Verification items for the finished model (mm, model axes). Round coordinates to 2 decimals unless told otherwise and drop trailing zeros. Loops run counter-clockwise (first coordinate to the right, second up) from the corner with the lowest first, then second, coordinate; pieces in that order, holes last. Notation, with made-up numbers: M 29.5,74 L 63.5,74 A28 cw 63.5,102 Z; hole C 29.5,34 d8. An arc over 180 degrees is marked long. One line per item, written item: value.
Autodesk Fusion 360 part; units mm, degrees
sketch "Sketch1" plane through (0, 0, 0) normal (0, 0, 1) x (1, 0, 0)
  circle A0 centre (0, 0) radius 200
  dimension "d1" = 400
extrude "Extrude1" add sketch "Sketch1" along normal blind 250
sketch "Sketch2" plane through (0, 0, 250) normal (0, 0, 1) x (-1, 0, 0)
  circle A0 centre (0, 0) radius 200
  circle A1 centre (0, 0) radius 25
  dimension "d4" = 50
extrude "Extrude2" cut sketch "Sketch2" against normal blind 75 contours A1
fillet "Fillet1" radius 25 1 edges at (-186.4655, -72.3231, 250)
scale "Scale1" factor 2.5 about (0, 0, 0) bodies 1
(1) Mould release check, pull along Y, two halves, no side actions. Record for faces 1 (the face through (91, 6, 625)), 2 (the face through (1, -1, 437.5)), 3 (the face through (62.44, -2.75, 532.56)), 4 (the face through (-499.516, -21.984, 277.312)): +Y half, -Y half, draft (parallel to the pull), parting line (faces both ways), or undercut.
Completed:
face 1: draft
face 2: undercut
face 3: undercut
face 4: parting line
(2) Thickness scan on L1, parallel to Y at x = 0, z = 486.5; L2, parallel to Y at x = 0, z = 433; L3, parallel to Z at x = -272, y = -344.5. Record the ranges inside material, lowest first. Write a range as from..to.
Completed:
L1: y = -500..-62.5, 62.5..500
L2: y = -500..500
L3: z = 0..624.98
(3) Sectioned sample at C-C on z = 205. Enter the section's corners in (x, y), and give its area (3 significant figures).
Completed:
outline: C 0,0 d1000
area: 785,000 mm^2
(4) Sectioned sample at A-A on x = 0. Enter the section's corners in (y, z).
Completed:
outline: M -500,0 L 500,0 L 500,562.5 A62.5 ccw 437.5,625 L 62.5,625 L 62.5,437.5 L -62.5,437.5 L -62.5,625 L -437.5,625 A62.5 ccw -500,562.5 Z
(5) Depth check by flat-ended pin: pin 1 Ø12 at (x, z) = (272.5, 452) entering from +Y; pin 2 Ø10 at (x, z) = (-359, 200) entering from +Y. Enter the tip coordinate at first touch or a pass-through.
Completed:
pin 1: stops at y = 423.06
pin 2: stops at y = 353.11
